from build123d import *

# Parameters (mm, degrees)
F0_R     = 1.5
F1_DEPTH = 13.5
F2_DEPTH = 2.5
F3_DEPTH = 2.5
F4_R     = 4
F5_DEPTH = 25


with BuildPart() as f1:
    # F0 (on Top) → F1 (new body)
    with BuildSketch(Plane.XY):
        with BuildLine():
            ThreePointArc((30.5, 0), (34, -3.5), (37.5, 0))
            ThreePointArc((37.5, 0), (34, 3.5), (30.5, 0))
        make_face()
        with BuildLine():
            ThreePointArc((35.5, 0), (34, -1.5), (32.5, 0))
            ThreePointArc((32.5, 0), (34, 1.5), (35.5, 0))
        make_face(mode=Mode.SUBTRACT)
        with BuildLine():
            ThreePointArc((-30.5, 0), (-34, 3.5), (-37.5, 0))
            ThreePointArc((-37.5, 0), (-34, -3.5), (-30.5, 0))
        make_face()
        with Locations((-34, 0)):
            Circle(F0_R, mode=Mode.SUBTRACT)
    extrude(amount=F1_DEPTH)

    # F0 (on Top) → F2 (join)
    with BuildSketch(Plane.XY):
        with BuildLine():
            ThreePointArc((30.5, 0), (34, 3.5), (37.5, 0))
            Line((37.5, 0), (37.5, 7.5))
            Line((37.5, 7.5), (-37.5, 7.5))
            Line((-37.5, 7.5), (-37.5, 0))
            ThreePointArc((-37.5, 0), (-34, 3.5), (-30.5, 0))
            Line((-30.5, 0), (0, 0))
            Line((0, 0), (30.5, 0))
        make_face()
    extrude(amount=F2_DEPTH)

    # F0 (on Top) → F3 (join)
    with BuildSketch(Plane.XY):
        with BuildLine():
            Line((-37.5, -7.5), (37.5, -7.5))
            Line((37.5, -7.5), (37.5, 0))
            ThreePointArc((37.5, 0), (34, -3.5), (30.5, 0))
            Line((30.5, 0), (0, 0))
            Line((0, 0), (-30.5, 0))
            ThreePointArc((-30.5, 0), (-34, -3.5), (-37.5, 0))
            Line((-37.5, 0), (-37.5, -7.5))
        make_face()
    extrude(amount=F3_DEPTH)

    # F4 (on Top) → F5 (cut)
    with BuildSketch(Plane.XY):
        Circle(F4_R)
    extrude(amount=F5_DEPTH, mode=Mode.SUBTRACT)


solid = f1.part
Check sheet for the modelled part. Datum: model origin and axes. Units: mm. A direction names the side the tool comes from. Round coordinates to 2 decimals unless told otherwise and drop trailing zeros. Loops run counter-clockwise (first coordinate to the right, second up) from the corner with the lowest first, then second, coordinate; pieces in that order, holes last. Notation, with made-up numbers: (69, 16) -> (89, 16) arc R23 cw to (89, 29) -> close; hole circle Ø5 at (-26.75, 74). An arc over 180 degrees is marked (long way). Put each result on its own line as item: value. Start each with the question number.
1. Section check B-B (z = 6.5). Enter the section's corners in (x, y).
2. Scan lines: probe 1 along Y at (x, z) = (34, 4.25); probe 2 along X at (y, z) = (1, 5.5); probe 3 along Y at (x, z) = (0, 1.55). Record each from-to range of solid material in increasing order.
3. Access from +Z, -Z, +X, -X, +Y, -Y to the whole of each face (thin tool, end or side, straight path). Record for faces 1 (the face through (-31.42, -2.365, 7.923)), 2 (the face through (34, -2, 13.5)).
4. Draft check along X on faces 3 (the face through (37.5, 0, 1)), 4 (the face through (35.2, -0.9, 6.7)), 5 (the face through (1, 7.5, 1)). Enter one of: +X half, -X half, draft (parallel to the pull), parting line (faces both ways), or undercut.
5. Section check A-A (x = 0). Enter the section's corners in (y, z).
6. Gauge pin test, flat ends, axial feed: pin 1 (4 mm diameter, centred on x = -34, y = 0, fed in from -Z); pin 2 (8 mm diameter, centred on x = -2, y = 0.5, fed in from +Z). Record the tip position at first contact, or that the pin passes through.
7. Section check C-C (x = -34). Enter the section's corners in (y, z).
8. Section check D-D (y = -6.5). Enter the section's corners in (x, z).
Findings:
1. outline: circle Ø7 at (-34, 0); circle Ø7 at (34, 0); hole circle Ø3 at (-34, 0); hole circle Ø3 at (34, 0)
2. probe 1: y = -3.5 to -1.5, 1.5 to 3.5
2. probe 2: x = -37.35 to -35.12, -32.88 to -30.65, 30.65 to 32.88, 35.12 to 37.35
2. probe 3: y = -7.5 to -4, 4 to 7.5
3. face 1: +Z
3. face 2: +Z, +X, -X, +Y, -Y
4. face 3: +X half
4. face 4: undercut
4. face 5: draft
5. outline: (-7.5, 0) -> (-4, 0) -> (-4, 2.5) -> (-7.5, 2.5) -> close; (4, 0) -> (7.5, 0) -> (7.5, 2.5) -> (4, 2.5) -> close
6. pin 1: stops at z = 0
6. pin 2: stops at z = 2.5
7. outline: (-7.5, 0) -> (-1.5, 0) -> (-1.5, 13.5) -> (-3.5, 13.5) -> (-3.5, 2.5) -> (-7.5, 2.5) -> close; (1.5, 0) -> (7.5, 0) -> (7.5, 2.5) -> (3.5, 2.5) -> (3.5, 13.5) -> (1.5, 13.5) -> close
8. outline: (-37.5, 0) -> (37.5, 0) -> (37.5, 2.5) -> (-37.5, 2.5) -> close
